```python
from build123d import *

# Parameters (mm, degrees)
BOSS_EXTRU_1_DEPTH      = 5
ESQUISSE2_W             = 130
ESQUISSE2_H             = 5
ENL_V_MAT_EXTRU_1_DEPTH = 5
ESQUISSE3_W             = 140
ESQUISSE3_H             = 5
BOSS_EXTRU_2_DEPTH      = 5


with BuildPart() as part:
    # Esquisse1 → Boss.-Extru.1 (new body)
    with BuildSketch(Plane.XY):
        Polygon((-83.248069132, -165.097223543), (-83.248069132, -160.097223543), (-88.248069132, -160.097223543), (-88.248069132, -150.097223543), (-83.248069132, -150.097223543), (-83.248069132, -140.097223543), (-88.248069132, -140.097223543), (-88.248069132, -130.097223543), (-83.248069132, -130.097223543), (-83.248069132, -120.097223543), (-88.248069132, -120.097223543), (-88.248069132, -110.097223543), (-83.248069132, -110.097223543), (-83.248069132, -100.097223543), (-88.248069132, -100.097223543), (-88.248069132, -90.097223543), (-83.248069132, -90.097223543), (-83.248069132, -85.097223543), (66.751930868, -85.097223543), (66.751930868, -90.097223543), (71.751930868, -90.097223543), (71.751930868, -100.097223543), (66.751930868, -100.097223543), (66.751930868, -110.097223543), (71.751930868, -110.097223543), (71.751930868, -120.097223543), (66.751930868, -120.097223543), (66.751930868, -130.097223543), (71.751930868, -130.097223543), (71.751930868, -140.097223543), (66.751930868, -140.097223543), (66.751930868, -150.097223543), (71.751930868, -150.097223543), (71.751930868, -160.097223543), (66.751930868, -160.097223543), (66.751930868, -165.097223543), align=None)
    extrude(amount=BOSS_EXTRU_1_DEPTH)

    # Esquisse2 → Enlèv. mat.-Extru.1 (cut)
    with BuildSketch(Plane.XY.offset(5)):
        with Locations((-8.248069132, -87.597223543)):
            Rectangle(ESQUISSE2_W, ESQUISSE2_H)
    extrude(amount=-ENL_V_MAT_EXTRU_1_DEPTH, mode=Mode.SUBTRACT)

    # Esquisse3 → Boss.-Extru.2 (add)
    with BuildSketch(Plane.XY.offset(5)):
        with Locations((-8.248069132, -167.597223543)):
            Rectangle(ESQUISSE3_W, ESQUISSE3_H)
    extrude(amount=-BOSS_EXTRU_2_DEPTH)


solid = part.part
```
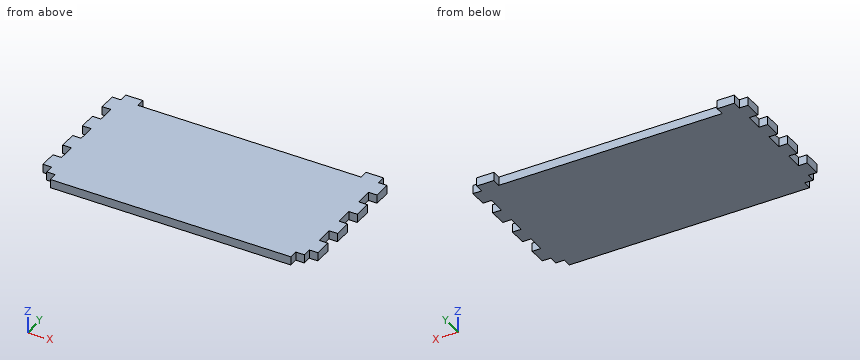
Could you check a few things on this model? Use its own coordinates, in mm. Round coordinates to 2 decimals unless told otherwise and drop trailing zeros. Order: outer loops, then holes, each group sorted by start corner. A loop starts at its lowest first (then second) coordinate and runs counter-clockwise, first axis right, second up. Notation, with made-up numbers: (47, 25) -> (63, 25) arc R7 cw to (63, 30) -> close; hole circle Ø10 at (-1, -34.75). An arc over 180 degrees is marked (long way). One line per question, with ' | ' between items.
Q1. If I drill on line 1 (Y direction, x = -35.5, z = 2.6); line 2 (X direction, y = -126, z = 0.75); line 3 (Y direction, x = -79, z = 1.4), over which ranges is the centre line in solid material (lowest first)? Write a range as from..to.
Computed values:
line 1: -170.1..-90.1 | line 2: -83.25..66.75 | line 3: -165.1..-85.1
Q2. If we section it at A-A on x = 34: Write out the boundary of the cut face in (y, z).
Computed values:
outline: (-170.1, 0) -> (-90.1, 0) -> (-90.1, 5) -> (-170.1, 5) -> close
Q3. I'm going to push flat-ended pins straight in: pin 1 (2.5 mm diameter, centred on y = -106, z = 2.5, fed in from +X); pin 2 (2.5 mm diameter, centred on y = -88, z = 2.5, fed in from -X); pin 3 (1.5 mm diameter, centred on x = 68.5, z = 2.5, fed in from +Y); pin 4 (1 mm diameter, centred on x = -8, y = -111.5, fed in from -Z). Where does each tip first touch, or does it pass through?
Computed values:
pin 1: x = 66.75 | pin 2: x = -83.25 | pin 3: y = -90.1 | pin 4: z = 0
